The model under review builds one solid part; all positions refer to its coordinate system, in mm. Coordinates: 2 decimals unless noted, no trailing zeros. Order: outer loops, then holes, each group sorted by start corner. A loop starts at its lowest first (then second) coordinate and runs counter-clockwise, first axis right, second up. Notation, with made-up numbers: M 77,83.25 L 134,83.25 A21 ccw 134,115.25 Z; hole C -9,28 d5. An arc over 180 degrees is marked long. Answer in a Markdown table with one row per item.
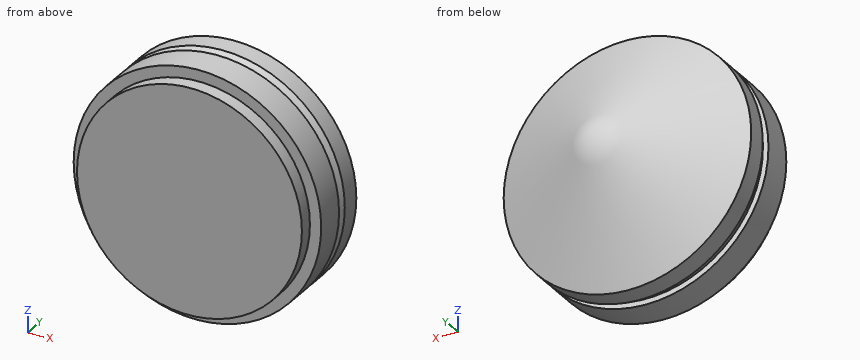
from build123d import *

# Parameters (mm, degrees)
SKETCH8_R           = 5.52
BOSS_EXTRUDE2_DEPTH = 0.7


with BuildPart() as part:
    # Sketch7 → Revolve1 (revolve)
    with BuildSketch(Plane.XY):
        Polygon((0, 55.134065354), (0, 48.724836522), (-6.075, 48.724836522), (-6.075, 50.284836522), (-5.8, 50.284836522), (-6.075, 50.784836522), (-6.075, 51.792815354), align=None)
    revolve(axis=Axis((0, 55.134065354, 0), (0, -1, 0)))

    # Sketch8 → Boss-Extrude2 (add)
    with BuildSketch(Plane.XZ.offset(-48.724836522)):
        Circle(SKETCH8_R)
    extrude(amount=BOSS_EXTRUDE2_DEPTH)


solid = part.part
(1) To check wall thickness, follow line 1 (X direction, y = 49, z = 0.5); line 2 (Y direction, x = -1.25, z = 5.5); line 3 (X direction, y = 51, z = 2). State the ranges of each line that lie inside material, in increasing order. Write a range as [from, to].
Report:
| item | result |
|---|---|
| line 1 | [-6.05, 6.05] |
| line 2 | [48.72, 52.03] |
| line 3 | [-5.74, 5.74] |
(2) Take a section at A-A (y = 49.5). Write out the cut boundary in (x, z) (3 decimals).
Report:
| item | result |
|---|---|
| outline | C 0,0 d12.15 |
(3) Insertion check: P1, Ø2, axis at y = 53.5, z = 1.5, coming from the -X side; P2, Ø2, axis at x = -1, z = 3, coming from the +Y side; P3, Ø1, axis at x = -4, y = 50, coming from the -Z side; P4, Ø6, axis at x = 1.5, z = -2.5, coming from the +Y side. Each pin has a flat end and moves straight along its axis. Give the tip position at first contact, or say it passes through.
Report:
| item | result |
|---|---|
| P1 | x = -4.57 |
| P2 | y = 53.94 |
| P3 | z = -4.97 |
| P4 | y = 55.13 |
(4) Take a section at B-B (y = 53). Write out the cut boundary in (x, z).
Report:
| item | result |
|---|---|
| outline | C 0,0 d7.76 |
